from build123d import *

# Parameters (mm, degrees)
F0_R     = 3.175
F1_DEPTH = 3.048


# Not quite as in the source:
# - a feature names something its author has since deleted; it is built from what else it names


with BuildPart() as f1:
    # F0 (on Front) → F1 (new body)
    with BuildSketch(Plane.XZ):
        with BuildLine():
            ThreePointArc((-25.2277835988, 89.1991540504), (-22.4379756896, 82.4639619596), (-15.7027835988, 79.6741540504))
            ThreePointArc((-15.7027835988, 79.6741540504), (-8.967591508, 82.4639619596), (-6.1777835988, 89.1991540504))
            ThreePointArc((-6.1777835988, 89.1991540504), (-15.7027835988, 98.7241540504), (-25.2277835988, 89.1991540504))
        make_face()
        with BuildLine():
            ThreePointArc((-12.5277835988, 89.1991540504), (-13.4577195686, 86.9540900201), (-15.7027835988, 86.0241540504))
            ThreePointArc((-15.7027835988, 86.0241540504), (-17.9478476291, 91.4442180807), (-12.5277835988, 89.1991540504))
        make_face(mode=Mode.SUBTRACT)
        with BuildLine():
            ThreePointArc((-6.1777835988, 89.1991540504), (-8.967591508, 82.4639619596), (-15.7027835988, 79.6741540504))
            Line((-15.7027835988, 79.6741540504), (-15.7027835988, 74.7860969014))
            Line((-15.7027835988, 74.7860969014), (-15.7027835988, 54.2741540504))
            ThreePointArc((-15.7027835988, 54.2741540504), (-5.7978377346, 50.8051071547), (-0.2218016911, 41.9140970332))
            Line((-0.2218016911, 41.9140970332), (-6.1777835988, 89.1991540504))
        make_face()
        with BuildLine():
            Line((-15.7027835988, 74.7860969014), (-15.7027835988, 79.6741540504))
            ThreePointArc((-15.7027835988, 79.6741540504), (-22.4379756896, 82.4639619596), (-25.2277835988, 89.1991540504))
            Line((-25.2277835988, 89.1991540504), (-31.1837655066, 41.9140970332))
            ThreePointArc((-31.1837655066, 41.9140970332), (-25.6077294631, 50.8051071547), (-15.7027835988, 54.2741540504))
            Line((-15.7027835988, 54.2741540504), (-15.7027835988, 74.7860969014))
        make_face()
        with Locations((-18.8777835988, 74.7860969014)):
            Circle(F0_R, mode=Mode.SUBTRACT)
        with BuildLine():
            ThreePointArc((-0.2218016911, 41.9140970332), (-5.7978377346, 50.8051071547), (-15.7027835988, 54.2741540504))
            Line((-15.7027835988, 54.2741540504), (-15.7027835988, 41.5741540504))
            ThreePointArc((-15.7027835988, 41.5741540504), (-13.4577195686, 40.6442180807), (-12.5277835988, 38.3991540504))
            ThreePointArc((-12.5277835988, 38.3991540504), (-13.4577195686, 36.1540900201), (-15.7027835988, 35.2241540504))
            Line((-15.7027835988, 35.2241540504), (-15.7027835988, 22.5241540504))
            ThreePointArc((-15.7027835988, 22.5241540504), (-5.8006414211, 25.990962994), (-0.2233918497, 34.8772148011))
            Line((-0.2233918497, 34.8772148011), (0.1662860895, 38.8330344781))
            Line((0.1662860895, 38.8330344781), (-0.2218016911, 41.9140970332))
        make_face()
        with BuildLine():
            Line((-15.7027835988, 41.5741540504), (-15.7027835988, 54.2741540504))
            ThreePointArc((-15.7027835988, 54.2741540504), (-25.6077294631, 50.8051071547), (-31.1837655066, 41.9140970332))
            Line((-31.1837655066, 41.9140970332), (-31.5718532872, 38.8330344781))
            Line((-31.5718532872, 38.8330344781), (-31.182175348, 34.8772148011))
            ThreePointArc((-31.182175348, 34.8772148011), (-25.6049257766, 25.990962994), (-15.7027835988, 22.5241540504))
            Line((-15.7027835988, 22.5241540504), (-15.7027835988, 35.2241540504))
            ThreePointArc((-15.7027835988, 35.2241540504), (-18.8777835988, 38.3991540504), (-15.7027835988, 41.5741540504))
        make_face()
        with BuildLine():
            Line((-31.5718532872, 38.8330344781), (-31.1837655066, 41.9140970332))
            ThreePointArc((-31.1837655066, 41.9140970332), (-31.4533286811, 40.3830780946), (-31.5718532872, 38.8330344781))
        make_face()
        with BuildLine():
            ThreePointArc((0.1662860895, 38.8330344781), (0.0477614834, 40.3830780946), (-0.2218016911, 41.9140970332))
            Line((-0.2218016911, 41.9140970332), (0.1662860895, 38.8330344781))
        make_face()
        with BuildLine():
            Line((-31.182175348, 34.8772148011), (-31.5718532872, 38.8330344781))
            ThreePointArc((-31.5718532872, 38.8330344781), (-31.5013163141, 36.8428799596), (-31.182175348, 34.8772148011))
        make_face()
        with BuildLine():
            ThreePointArc((0.1722164012, 38.3991540504), (0.170733754, 38.6161145273), (0.1662860895, 38.8330344781))
            Line((0.1662860895, 38.8330344781), (-0.2233918497, 34.8772148011))
            ThreePointArc((-0.2233918497, 34.8772148011), (0.0730043216, 36.6271098943), (0.1722164012, 38.3991540504))
        make_face()
        with BuildLine():
            ThreePointArc((-15.7027835988, 22.5241540504), (-25.6049257766, 25.990962994), (-31.182175348, 34.8772148011))
            Line((-31.182175348, 34.8772148011), (-25.181903228, -26.034610404))
            ThreePointArc((-25.181903228, -26.034610404), (-22.7603940807, -18.7043031892), (-15.7027835988, -15.5758459496))
            Line((-15.7027835988, -15.5758459496), (-15.7027835988, 22.5241540504))
        make_face()
        with BuildLine():
            Line((-4.7578265809, -11.1541468152), (-0.2233918497, 34.8772148011))
            ThreePointArc((-0.2233918497, 34.8772148011), (-5.8006414211, 25.990962994), (-15.7027835988, 22.5241540504))
            Line((-15.7027835988, 22.5241540504), (-15.7027835988, -15.5758459496))
            ThreePointArc((-15.7027835988, -15.5758459496), (-8.967591508, -18.3656538588), (-6.1777835988, -25.1008459496))
            ThreePointArc((-6.1777835988, -25.1008459496), (-7.8814722685, -30.5370867531), (-12.3830778926, -34.0286216538))
            Line((-12.3830778926, -34.0286216538), (21.5012593326, -34.0286216538))
            ThreePointArc((21.5012593326, -34.0286216538), (17.8308984551, -25.2118628548), (25.291047986, -19.2492330938))
            Line((25.291047986, -19.2492330938), (3.3830391656, -19.8804312387))
            ThreePointArc((3.3830391656, -19.8804312387), (-2.6591751738, -17.3567899438), (-4.7578265809, -11.1541468152))
        make_face()
        with BuildLine():
            ThreePointArc((-15.7027835988, -15.5758459496), (-22.7603940807, -18.7043031892), (-25.181903228, -26.034610404))
            ThreePointArc((-25.181903228, -26.034610404), (-23.2478837609, -30.9143722928), (-19.022489305, -34.0286216538))
            Line((-19.022489305, -34.0286216538), (-12.3830778926, -34.0286216538))
            ThreePointArc((-12.3830778926, -34.0286216538), (-7.8814722685, -30.5370867531), (-6.1777835988, -25.1008459496))
            ThreePointArc((-6.1777835988, -25.1008459496), (-8.967591508, -18.3656538588), (-15.7027835988, -15.5758459496))
        make_face()
        with BuildLine():
            ThreePointArc((-12.5277835988, -25.1008459496), (-17.9478476291, -27.3459099799), (-15.7027835988, -21.9258459496))
            ThreePointArc((-15.7027835988, -21.9258459496), (-13.4577195686, -22.8557819193), (-12.5277835988, -25.1008459496))
        make_face(mode=Mode.SUBTRACT)
        with BuildLine():
            Line((-12.3830778926, -34.0286216538), (-19.022489305, -34.0286216538))
            ThreePointArc((-19.022489305, -34.0286216538), (-15.7027835988, -34.6258459496), (-12.3830778926, -34.0286216538))
        make_face()
        with BuildLine():
            ThreePointArc((33.4571426277, -27.1834407253), (31.0508918664, -21.4905339011), (25.291047986, -19.2492330938))
            ThreePointArc((25.291047986, -19.2492330938), (17.8308984551, -25.2118628548), (21.5012593326, -34.0286216538))
            ThreePointArc((21.5012593326, -34.0286216538), (29.4634979017, -34.0718303649), (33.4571426277, -27.1834407253))
        make_face()
        with Locations((25.5196426277, -27.1834407253)):
            Circle(F0_R, mode=Mode.SUBTRACT)
    extrude(amount=F1_DEPTH)


solid = f1.part
Read the model definition and answer for the solid it produces. Units are mm, in the model's axes. A direction names the side the tool comes from. Give positions to 0.01 mm unless a question says otherwise; leave off trailing zeros. Loops run counter-clockwise (first coordinate to the right, second up) from the corner with the lowest first, then second, coordinate; pieces in that order, holes last. Notation, with made-up numbers: (80.25, 6) -> (100.25, 6) arc R30 ccw to (100.25, 42) -> close; hole circle Ø9 at (73.5, -15). An arc over 180 degrees is marked (long way). Use a Markdown table: item, result.
Q1. Find the intervals of material crossed by line 1 along Z through (x, y) = (-18, -1.1); line 2 along Z through (x, y) = (-14, -0.1); line 3 along Z through (x, y) = (-17, -1.15), in increasing order.
Solved:
| item | result |
|---|---|
| line 1 | z = -34.34 to -27.29, -22.91 to 36.21, 40.59 to 71.73, 77.84 to 87.01, 91.39 to 98.44 |
| line 2 | z = -34.47 to -27.78, -22.42 to 35.72, 41.08 to 86.52, 91.88 to 98.57 |
| line 3 | z = -34.54 to -28, -22.2 to 35.5, 41.3 to 72.23, 77.35 to 86.3, 92.1 to 98.64 |
Q2. Each of these flat-tipped pins is pushed along its axis until it touches: pin 1 (7.5 mm diameter, centred on x = -18.88, z = 74.79, fed in from +Y); pin 2 (1.5 mm diameter, centred on x = -7.5, y = -2.5, fed in from -Z); pin 3 (1.5 mm diameter, centred on y = -2.5, z = 9, fed in from -X); pin 4 (5.5 mm diameter, centred on x = 25.52, z = -27.18, fed in from +Y). Where does it stop, or does it pass through?
Solved:
| item | result |
|---|---|
| pin 1 | stops at y = 0 |
| pin 2 | stops at z = -34.03 |
| pin 3 | stops at x = -28.71 |
| pin 4 | passes through |
Q3. Section C-C, the plane x = 14.5 is taken. Determine the outline of the cut face in (y, z).
Solved:
| item | result |
|---|---|
| outline | (-3.05, -34.03) -> (0, -34.03) -> (0, -19.56) -> (-3.05, -19.56) -> close |
Q4. A tool of negligible diameter and unlimited length cuts with its end or side. For faces 1 (the face through (-2.522, -1.503, 11.539)), 2 (the face through (-2.59, -1.5, -17.43)), 3 (the face through (4, -2, -34.029)), from which of +Z, -Z, +X, -X, +Y, -Y can it reach the whole face along a straight path? Write none if from no direction.
Solved:
| item | result |
|---|---|
| face 1 | +X, +Y, -Y |
| face 2 | +Y, -Y |
| face 3 | -Z, +Y, -Y |
Q5. Section D-D, the plane z = 59.5 is taken. Determine the outline of the cut face in (x, y), then the cut area to 3 significant figures.
Solved:
| item | result |
|---|---|
| outline | (-28.97, -3.05) -> (-2.44, -3.05) -> (-2.44, 0) -> (-28.97, 0) -> close |
| area | 80.9 mm^2 |
Q6. Section A-A, the plane z = 36.5 is taken. Determine the outline of the cut face in (x, y).
Solved:
| item | result |
|---|---|
| outline | (-31.46, -3.05) -> (-18.25, -3.05) -> (-18.25, 0) -> (-31.46, 0) -> close; (-13.16, -3.05) -> (0.06, -3.05) -> (0.06, 0) -> (-13.16, 0) -> close |
Q7. Section B-B, the plane y = -1.5 is taken. Count the separate pieces of the cut face and the enclosed holes in it, then the cut area to 3 significant figures.
Solved:
| item | result |
|---|---|
| separate pieces | 1 |
| enclosed holes | 5 |
| area | 3,620 mm^2 |
Q8. Determine the mould class of faces 4 (the face through (-14, 0, 33)), 5 (the face through (24.831, -1.503, -30.283)), 6 (the face through (-28.164, -1.503, 65.888)) for opening direction X: pulls with the +X half, pulls with the -X half, needs draft (parallel to the pull), parting line crosses it, or undercut.
Solved:
| item | result |
|---|---|
| face 4 | needs draft |
| face 5 | undercut |
| face 6 | pulls with the -X half |
